Source: CAD feature listing. Evaluate the final solid. Frame: model axes, mm. A direction names the side the tool comes from. Coordinates: 2 decimals unless noted, no trailing zeros. Order: outer loops, then holes, each group sorted by start corner. A loop starts at its lowest first (then second) coordinate and runs counter-clockwise, first axis right, second up. Notation, with made-up numbers: (69, 75.25) -> (128, 75.25) arc R19 ccw to (128, 102.25) -> close; hole circle Ø10 at (33, 70). An arc over 180 degrees is marked (long way). Put each result on its own line as item: value.
from build123d import *

# Parameters (mm, degrees)
SKETCH_1_W          = 50
SKETCH_1_H          = 50
SKETCH_1_W_2        = 42
SKETCH_1_H_2        = 42
EXTRUDE_1_DEPTH     = 750
SKETCH_2_R          = 6
CUT_EXTRUDE_1_DEPTH = 753.080447825


with BuildPart() as part:
    # 草图1 → 凸台-拉伸1 (new, symmetric)
    with BuildSketch(Plane.XY):
        Rectangle(SKETCH_1_W, SKETCH_1_H)
        Rectangle(SKETCH_1_W_2, SKETCH_1_H_2, mode=Mode.SUBTRACT)
    extrude(amount=EXTRUDE_1_DEPTH, both=True)

    # 草图2 → 切除-拉伸1 (cut, through all)
    with BuildSketch(Plane(origin=(0, 25, 0), x_dir=(1, 0, 0), z_dir=(0, 1, 0))):
        with Locations(Location((0, 0, 0), (0, 0, 270))):
            Circle(SKETCH_2_R)
    extrude(amount=-CUT_EXTRUDE_1_DEPTH, mode=Mode.SUBTRACT)


solid = part.part
1. Set-up query: faces 1 (the flat face through (0, 25, 10)), 2 (the flat face through (-21, 0, 10)). Return all of +Z, -Z, +X, -X, +Y, -Y with unobstructed straight access to the full face (end or side cutting, diameter ignored); none if empty.
Numbers:
face 1: +Z, -Z, +X, -X, +Y
face 2: +Z, -Z
2. Ray query, line 1 along X through (y, z) = (-23.2, 0); line 2 along X through (y, z) = (12, 159.5). Return the intervals inside material, ascending.
Numbers:
line 1: x = -25 to -6, 6 to 25
line 2: x = -25 to -21, 21 to 25
3. Pull-direction query (Y, two-part tool) for faces 3 (the flat face through (-23, 0, -750)), 4 (the flat face through (0, 21, 10)), 5 (the flat face through (0, -25, 10)); classes: pulls with the +Y half, pulls with the -Y half, needs draft (parallel to the pull), parting line crosses it, or undercut.
Numbers:
face 3: needs draft
face 4: undercut
face 5: pulls with the -Y half
4. Cut plane A-A on z = 204. Output: boundary loops of the cut face in (x, y).
Numbers:
outline: (-25, -25) -> (25, -25) -> (25, 25) -> (-25, 25) -> close; hole (-21, -21) -> (21, -21) -> (21, 21) -> (-21, 21) -> close
5. Cut plane B-B on y = -4. Output: boundary loops of the cut face in (x, z).
Numbers:
outline: (-25, -750) -> (-21, -750) -> (-21, 750) -> (-25, 750) -> close; (21, -750) -> (25, -750) -> (25, 750) -> (21, 750) -> close
6. First-contact query: pin 1 (9.5 mm diameter, centred on x = 0, z = 0, fed in from +Y). Flat tip, straight axial feed; report the tip coordinate or a pass-through.
Numbers:
pin 1: passes through
